```python
from build123d import *

# Parameters (mm, degrees)
F0_W      = 68.4
F0_H      = 31.2
F1_DEPTH  = 9.2
F3_DEPTH  = 7.6
F4_R      = 2
F5_R      = 2
F6_R      = 2
F7_R      = 2.5
F8_DEPTH  = 5
F10_D     = 2
F10_DEPTH = 4
F10_TIP   = 0.600860619
F12_D     = 2
F12_DEPTH = 4
F12_TIP   = 0.600860619
F13_R     = 2.2
F14_DEPTH = 1.601
F15_SIZE  = 0.5


with BuildPart() as f1:
    # F0 (on Front) → F1 (new body)
    with BuildSketch(Plane.XZ):
        Rectangle(F0_W, F0_H)
    extrude(amount=F1_DEPTH)

    # F2 (on face) → F3 (cut)
    with BuildSketch(Plane.XZ.offset(9.2)):
        with BuildLine():
            ThreePointArc((32.6, 13), (30.8928932188, 12.2928932188), (31.6, 14))
            Line((31.6, 14), (-31.6, 14))
            ThreePointArc((-31.6, 14), (-30.8928932188, 13.7071067812), (-30.6, 13))
            ThreePointArc((-30.6, 13), (-31.6, 12), (-32.6, 13))
            Line((-32.6, 13), (-32.6, -12))
            Line((-32.6, -12), (-34.2, -12))
            Line((-34.2, -12), (-34.2, -15.6))
            Line((-34.2, -15.6), (34.2, -15.6))
            Line((34.2, -15.6), (34.2, -12))
            Line((34.2, -12), (32.6, -12))
            Line((32.6, -12), (32.6, 13))
        make_face()
        with BuildLine():
            ThreePointArc((32.6, 13), (32.3071067812, 13.7071067812), (31.6, 14))
            ThreePointArc((31.6, 14), (30.8928932188, 12.2928932188), (32.6, 13))
        make_face()
        with BuildLine():
            ThreePointArc((-30.6, 13), (-30.8928932188, 13.7071067812), (-31.6, 14))
            ThreePointArc((-31.6, 14), (-32.3071067812, 13.7071067812), (-32.6, 13))
            ThreePointArc((-32.6, 13), (-31.6, 12), (-30.6, 13))
        make_face()
    extrude(amount=-F3_DEPTH, mode=Mode.SUBTRACT)

    # F4
    f4_edges = [f1.edges().sort_by_distance(p)[0] for p in [
        (34.2, -4.6, 15.6),
    ]]
    fillet(f4_edges, radius=F4_R)

    # F5
    f5_edges = [f1.edges().sort_by_distance(p)[0] for p in [
        (-34.2, -4.6, 15.6),
        (-34.2, -0.8, -15.6),
    ]]
    fillet(f5_edges, radius=F5_R)

    # F6
    f6_edges = [f1.edges().sort_by_distance(p)[0] for p in [
        (34.2, -0.8, -15.6),
    ]]
    fillet(f6_edges, radius=F6_R)

    # F7 (on face) → F8 (join)
    with BuildSketch(Plane.XZ.offset(1.6)):
        with Locations((-27, -2)):
            Circle(F7_R)
        with Locations((27, -2)):
            Circle(F7_R)
    extrude(amount=F8_DEPTH)

    # F10
    with Locations(Plane.XZ.offset(6.6)):
        with Locations((-27, -2)):
            Hole(F10_D / 2, depth=F10_DEPTH)
            with Locations((0, 0, -(F10_DEPTH + F10_TIP / 2))):  # 118° drill point
                Cone(0, F10_D / 2, F10_TIP, mode=Mode.SUBTRACT)

    # F12
    with Locations(Plane.XZ.offset(6.6)):
        with Locations((27, -2)):
            Hole(F12_D / 2, depth=F12_DEPTH)
            with Locations((0, 0, -(F12_DEPTH + F12_TIP / 2))):  # 118° drill point
                Cone(0, F12_D / 2, F12_TIP, mode=Mode.SUBTRACT)

    # F13 (on face) → F14 (cut, through all)
    with BuildSketch(Plane(origin=(32.6, 0, 0), x_dir=(0, -1, 0), z_dir=(-1, 0, 0))):
        with Locations((4.2, 8.6)):
            Circle(F13_R)
    extrude(amount=-F14_DEPTH, mode=Mode.SUBTRACT)

    # F15
    f15_edges = [f1.edges().sort_by_distance(p)[0] for p in [
        (34.2, -2, 8.6),
    ]]
    chamfer(f15_edges, length=F15_SIZE)


solid = f1.part
```
The listing builds one solid part. Answer for the finished solid, in the listing's coordinates (mm). A direction names the side the tool comes from. Coordinates: 2 decimals unless noted, no trailing zeros. Loops run counter-clockwise (first coordinate to the right, second up) from the corner with the lowest first, then second, coordinate; pieces in that order, holes last. Notation, with made-up numbers: M 57.5,56.25 L 72.5,56.25 A21 ccw 72.5,91.25 Z; hole C 56,23 d4. An arc over 180 degrees is marked long. Answer as a JSON object with one key per item and string values. Group by question number.
Item 1: Each of these flat-tipped pins is pushed along its axis until it touches: P1, Ø1.6, axis at x = 27, z = -2, coming from the -Y side; P2, Ø6, axis at x = 18.5, z = -2.5, coming from the -Y side; P3, Ø2.5, axis at x = 1, y = -5, coming from the -Z side. Where does it stop, or does it pass through?
Item 2: Section D-D (x = -13) is taken. Write down the section's boundary in (y, z), and give its area (3 significant figures).
Item 3: Which of the six approach directions +Z, -Z, +X, -X, +Y, -Y give full straight-line access (tool end or side, diameter ignored) to faces 4 (the face through (28, -6.6, -3)), 5 (the face through (33.142, -3.723, 6.452)), 6 (the face through (28, -5, -2))?
Item 4: Section B-B (z = 8.6) is taken. Write down the section's boundary in (x, y), and give its area (3 significant figures).
Item 5: Section C-C (z = 2) is taken. Write down the section's boundary in (x, y).
Item 6: Consider L1, parallel to Z at x = 27, y = -5.1; L2, parallel to X at y = -1.75, z = 4; L3, parallel to Y at x = 22, z = -5. Determine where each line is inside the solid, lowest interval first.
Item 7: Determine the mould class of faces 1 (the face through (33.6, -0.81, -15.03)), 2 (the face through (34.2, -5, 0)), 3 (the face through (-26, -5, -2)) for opening direction Z: +Z half, -Z half, draft (parallel to the pull), parting line (faces both ways), or undercut.
Item 8: Section A-A (y = -4.2) is taken. Write down the section's boundary in (x, z).
Solved:
{
 "1": {"P1": "stops at y = -2.48", "P2": "stops at y = -1.6", "P3": "stops at z = 14"},
 "2": {"outline": "M -9.2,14 L -1.6,14 L -1.6,-15.6 L 0,-15.6 L 0,15.6 L -9.2,15.6 Z", "area": "62.1 mm2"},
 "3": {"face 4": "-Z, -Y", "face 5": "+X", "face 6": "-Y"},
 "4": {"outline": "M -34.2,-9.2 L -32.6,-9.2 L -32.6,-1.6 L 32.6,-1.6 L 32.6,-2 L 33.7,-2 L 34.2,-1.5 L 34.2,0 L -34.2,0 Z; M 32.6,-9.2 L 34.2,-9.2 L 34.2,-6.9 L 33.7,-6.4 L 32.6,-6.4 Z", "area": "126 mm2"},
 "5": {"outline": "M -34.2,-9.2 L -32.6,-9.2 L -32.6,-1.6 L 32.6,-1.6 L 32.6,-9.2 L 34.2,-9.2 L 34.2,0 L -34.2,0 Z"},
 "6": {"L1": "z = -4.5 to -3, -1 to 0.5, 14 to 15.6", "L2": "x = -34.2 to -32.6, 32.6 to 34.2", "L3": "y = -1.6 to 0"},
 "7": {"face 1": "-Z half", "face 2": "draft", "face 3": "undercut"},
 "8": {"outline": "M -34.2,-12 L -32.6,-12 L -32.6,13 A1 cw -31.6,14 L 31.6,14 A1 cw 32.6,13 L 32.6,10.8 L 33.7,10.8 L 34.2,11.3 L 34.2,13.6 A2 ccw 32.2,15.6 L -32.2,15.6 A2 ccw -34.2,13.6 Z; C -27,-2 d5; C 27,-2 d5; M 32.6,-12 L 34.2,-12 L 34.2,5.9 L 33.7,6.4 L 32.6,6.4 Z; hole C -27,-2 d2; hole C 27,-2 d2"}
}
